```python
from build123d import *

# Parameters (mm, degrees)
SKIZZE1_R                       = 1.5
AUFSATZ_LINEAR_AUSTRAGEN1_DEPTH = 59
SKIZZE2_R                       = 10.5
AUFSATZ_LINEAR_AUSTRAGEN2_DEPTH = 2
SKIZZE3_R                       = 2.5
AUFSATZ_LINEAR_AUSTRAGEN3_DEPTH = 23
SCHNITT_LINEAR_AUSTRAGEN1_DEPTH = 15


with BuildPart() as part:
    # Skizze1 → Aufsatz-Linear austragen1 (new body)
    with BuildSketch(Plane.XY):
        Polygon((-17, -21), (17, -21), (21, -17), (21, 17), (17, 21), (-17, 21), (-21, 17), (-21, -17), align=None)
        with Locations((15.5, 15.5)):
            Circle(SKIZZE1_R, mode=Mode.SUBTRACT)
        with Locations((15.5, -15.5)):
            Circle(SKIZZE1_R, mode=Mode.SUBTRACT)
        with Locations((-15.5, -15.5)):
            Circle(SKIZZE1_R, mode=Mode.SUBTRACT)
        with Locations((-15.5, 15.5)):
            Circle(SKIZZE1_R, mode=Mode.SUBTRACT)
    extrude(amount=AUFSATZ_LINEAR_AUSTRAGEN1_DEPTH)

    # Skizze2 → Aufsatz-Linear austragen2 (add)
    with BuildSketch(Plane.XY.offset(59)):
        with Locations(Location((0, 0, 0), (0, 0, 180))):
            Circle(SKIZZE2_R)
    extrude(amount=AUFSATZ_LINEAR_AUSTRAGEN2_DEPTH)

    # Skizze3 → Aufsatz-Linear austragen3 (add)
    with BuildSketch(Plane.XY.offset(61)):
        Circle(SKIZZE3_R)
    extrude(amount=AUFSATZ_LINEAR_AUSTRAGEN3_DEPTH)

    # Skizze4 → Schnitt-Linear austragen1 (cut)
    with BuildSketch(Plane.XY.offset(84)):
        Polygon((-75.850602173, 2), (-1.5, 2), (1.5, 2), (75.850602173, 2), (75.850602173, 150.701204346), (-75.850602173, 150.701204346), align=None)
    extrude(amount=-SCHNITT_LINEAR_AUSTRAGEN1_DEPTH, mode=Mode.SUBTRACT)


solid = part.part
```
Build history of the part. All positions in model axes, mm. A direction names the side the tool comes from. Coordinates: 2 decimals unless noted, no trailing zeros. Order: outer loops, then holes, each group sorted by start corner. A loop starts at its lowest first (then second) coordinate and runs counter-clockwise, first axis right, second up. Notation, with made-up numbers: M 39,49 L 94,49 A34 cw 94,81 Z; hole C 4,78 d6. An arc over 180 degrees is marked long. One line per question, with ' | ' between items. Start each with the question number.
1. Cut at A-A (y = 15.5). Write the cut outline in (x, z), plus the area to 3 significant figures.
2. Tool access for faces 1 (the face through (-10, 5, 59)), 2 (the face through (0, 2, 77)), 3 (the face through (19, 19, 29)): list every direction of +Z, -Z, +X, -X, +Y, -Y with a clear straight run to the whole face (end or side of a thin tool).
3. Flat gauge pins, fed straight in: P1, Ø6.5, axis at x = 4, y = -4, coming from the +Z side; P2, Ø2.5, axis at x = 15.5, y = -15.5, coming from the +Z side; P3, Ø2, axis at x = 3, y = 9.5, coming from the +Z side; P4, Ø12, axis at y = -4.5, z = 71.5, coming from the +X side. Where does each tip first touch, or does it go through?
4. Mould opens along X. For faces 4 (the face through (14, -15.43, 29.09)), 5 (the face through (-10, -3.2, 60)), 6 (the face through (-19, -19, 29)), 7 (the face through (-17, -15.43, 29.09)) say: +X half, -X half, draft (parallel to the pull), parting line (faces both ways), or undercut.
5. Wall check: line 1 along Y through (x, z) = (-15.5, 23); line 2 along Y through (x, z) = (-15, 30); line 3 along Z through (x, y) = (11.5, -8.5). Give the ranges that are in metal, low to high. Write a range as [from, to].
6. Cut at C-C (z = 11.5). Write the cut outline in (x, y).
7. Cut at D-D (x = 0). Write the cut outline in (y, z).
The answers:
1) outline: M -21,0 L -17,0 L -17,59 L -21,59 Z; M -14,0 L 14,0 L 14,59 L -14,59 Z; M 17,0 L 21,0 L 21,59 L 17,59 Z | area: 2,120 mm2
2) face 1: +Z | face 2: +Z, +X, -X, +Y | face 3: +Z, -Z, +X, +Y
3) P1: stops at z = 84 | P2: passes through | P3: stops at z = 61 | P4: stops at x = 2.5
4) face 4: undercut | face 5: parting line | face 6: -X half | face 7: undercut
5) line 1: y = [-21, -17], [-14, 14], [17, 21] | line 2: y = [-21, -16.91], [-14.09, 14.09], [16.91, 21] | line 3: z = [0, 59]
6) outline: M -21,-17 L -17,-21 L 17,-21 L 21,-17 L 21,17 L 17,21 L -17,21 L -21,17 Z; hole C -15.5,-15.5 d3; hole C -15.5,15.5 d3; hole C 15.5,-15.5 d3; hole C 15.5,15.5 d3
7) outline: M -21,0 L 21,0 L 21,59 L 10.5,59 L 10.5,61 L 2.5,61 L 2.5,69 L 2,69 L 2,84 L -2.5,84 L -2.5,61 L -10.5,61 L -10.5,59 L -21,59 Z
